Autodesk Inventor part; units mm, degrees
ref_plane "YZ Plane" through (0, 0, 0) normal (1, 0, 0) x (0, 1, 0)
ref_plane "XZ Plane" through (0, 0, 0) normal (0, 1, 0) x (-1, 0, 0)
ref_plane "XY Plane" through (0, 0, 0) normal (0, 0, 1) x (1, 0, 0)
sketch "Sketch1" plane through (0, 0, 0) normal (0, 0, 1) x (1, 0, 0)
  circle A0 centre (57.1655, 18.417) radius 2.1
  circle A1 centre (12.7885, 12.5269) radius 2.1
  circle A2 centre (17.2869, -26.8107) radius 2.1
  circle A3 centre (-1.1004, -6.0436) radius 5
  line L0 (64.4194, 6.1067) -> (62.3371, -1.6056)
  line L1 (67.3095, 9.3686) -> (64.4194, 6.1067)
  ellipse E0 centre (57.1655, 18.417) end of major axis (47.0979, 27.5508) minor radius 11.51 (67.3095, 9.3686) -> (68.6853, 21.7358) ccw
  ellipse E1 centre (54.4602, 15.4351) end of major axis (43.6731, 3.5452) minor radius 13.5934 (68.6853, 21.7358) -> (59.3507, 30.2045) ccw
  ellipse E2 centre (57.1655, 18.417) end of major axis (47.0979, 27.5508) minor radius 11.51 (59.3507, 30.2045) -> (47.0214, 27.4655) ccw
  line L2 (36.5043, 15.5956) -> (47.0214, 27.4655)
  arc A4 (36.5043, 15.5956) -> (29.6862, 12.4398) centre (33.7853, 12.5269) ccw
  line L3 (16.8875, 12.4398) -> (29.6862, 12.4398)
  arc A5 (16.8875, 12.4398) -> (10.0695, 15.5956) centre (12.7885, 12.5269) ccw
  line L4 (10.0695, 15.5956) -> (-0.4476, 27.4655)
  ellipse E3 centre (-10.5917, 18.417) end of major axis (-0.5241, 27.5508) minor radius 11.51 (-0.4476, 27.4655) -> (-12.7769, 30.2045) ccw
  ellipse E4 centre (-7.8864, 15.4351) end of major axis (2.9006, 3.5452) minor radius 13.5934 (-12.7769, 30.2045) -> (-22.1115, 21.7358) ccw
  ellipse E5 centre (-10.5917, 18.417) end of major axis (-0.5241, 27.5508) minor radius 11.51 (-22.1115, 21.7358) -> (-20.7358, 9.3686) ccw
  line L5 (-20.7358, 9.3686) -> (-17.8456, 6.1067)
  line L6 (-17.8456, 6.1067) -> (-15.7633, -1.6056)
  line L7 (-15.7633, -1.6056) -> (-6.4546, -11.2249)
  line L8 (-6.4546, -11.2249) -> (1.9738, -21.6241)
  line L9 (1.9738, -21.6241) -> (9.6038, -24.7107)
  line L10 (9.6038, -24.7107) -> (14.4693, -29.7892)
  arc A6 (14.4693, -29.7892) -> (17.2869, -30.9107) centre (17.2869, -26.8107) ccw
  line L11 (17.2869, -30.9107) -> (29.2869, -30.9107)
  arc A7 (29.2869, -30.9107) -> (32.1045, -29.7892) centre (29.2869, -26.8107) ccw
  line L12 (36.97, -24.7107) -> (32.1045, -29.7892)
  line L13 (44.6, -21.6241) -> (36.97, -24.7107)
  line L14 (53.0284, -11.2249) -> (44.6, -21.6241)
  line L15 (62.3371, -1.6056) -> (53.0284, -11.2249)
  circle A8 centre (-10.5917, 18.417) radius 2.1
  circle A9 centre (47.6742, -6.0436) radius 5
  circle A10 centre (29.2869, -26.8107) radius 2.1
  circle A11 centre (33.7853, 12.5269) radius 2.1
  arc A12 (-51.3703, 45.0767) -> (97.4441, 45.0767) centre (23.0369, 31.7099) ccw construction
  arc A13 (51.5869, 99.9923) -> (-5.5131, 99.9923) centre (23.0369, 31.7099) ccw construction
  arc A14 (-50.582, -28.3339) -> (101.2571, -22.203) centre (23.0369, 31.7099) ccw construction
  line L16 (23.0369, 31.7099) -> (23.2869, -30.9107) construction
  line L17 (85.5258, 132.2899) -> (-39.4742, 132.2899)
  line L18 (-39.4742, 132.2899) -> (-39.4742, -63.2901)
  line L19 (-39.4742, -63.2901) -> (85.5258, -63.2901)
  line L20 (85.5258, -63.2901) -> (85.5258, 132.2899)
  line L21 (85.5258, 132.2899) -> (-39.4742, -63.2901) construction
  line L22 (-39.4742, 132.2899) -> (85.5258, -63.2901) construction
  point P0 (0, 0)
  point P1 (23.0258, 34.4999)
  dimension "d0" = 195.58
  dimension "d27" = 125
extrude "Extrusion1" add sketch "Sketch1" along normal blind 4 contours L0 L15 L14 L13 L12 A7 L11 A6 L10 L9 L8 L7 L6 L5 E5 E4 E3 L4 A5 L3 A4 L2 E2 E1 E0 L1 | L20 L19 L18 L17
sketch "Sketch2" plane through (0, 0, 4) normal (0, 0, 1) x (1, 0, 0)
  line L0 (-39.4742, 132.2899) -> (-39.4742, -63.2901)
  line L1 (-39.4742, -63.2901) -> (85.5258, -63.2901)
  line L2 (85.5258, -63.2901) -> (85.5258, 132.2899)
  line L3 (85.5258, 132.2899) -> (-39.4742, 132.2899)
  circle A0 centre (12.7885, 12.5269) radius 2.1
  circle A1 centre (33.7853, 12.5269) radius 2.1
  circle A2 centre (29.2869, -26.8107) radius 2.1
  circle A3 centre (47.6742, -6.0436) radius 5
  circle A4 centre (-10.5917, 18.417) radius 2.1
  circle A5 centre (-1.1004, -6.0436) radius 5
  circle A6 centre (17.2869, -26.8107) radius 2.1
  circle A7 centre (57.1655, 18.417) radius 2.1
  line L4 (85.5258, 132.2899) -> (-39.4742, 132.2899)
  line L5 (-39.4742, 132.2899) -> (-39.4742, 127.2899)
  line L6 (-39.4742, 127.2899) -> (85.5258, 127.2899)
  line L7 (85.5258, 127.2899) -> (85.5258, 132.2899)
  line L8 (52.5258, 127.2899) -> (-6.4742, 127.2899)
  line L9 (-6.4742, 127.2899) -> (-6.4742, 133.2899)
  line L10 (-6.4742, 133.2899) -> (52.5258, 133.2899)
  line L11 (52.5258, 133.2899) -> (52.5258, 127.2899)
  point P0 (0, 0)
  point P1 (-39.4742, 127.2899)
  point P2 (85.5258, 127.2899)
  dimension "d3" = 5
  dimension "d7" = 6
  dimension "d8" = 33
  dimension "d9" = 33
extrude "Extrusion2" add sketch "Sketch2" along normal blind 130 contours L3 L9 L6 L0 | L3 L11 L6 L9 | L3 L2 L6 L11
sketch "Sketch4" plane through (0, 0, 134) normal (0, 0, 1) x (1, 0, 0)
  line L0 (85.5258, 127.2899) -> (-39.4742, 127.2899)
  line L1 (-39.4742, 127.2899) -> (-39.4742, -63.2901)
  line L2 (-39.4742, -63.2901) -> (85.5258, -63.2901)
  line L3 (85.5258, -63.2901) -> (85.5258, 127.2899)
  circle A0 centre (12.7885, 12.5269) radius 2.1
  circle A1 centre (33.7853, 12.5269) radius 2.1
  circle A2 centre (29.2869, -26.8107) radius 2.1
  circle A3 centre (47.6742, -6.0436) radius 5
  circle A4 centre (-10.5917, 18.417) radius 2.1
  circle A5 centre (-1.1004, -6.0436) radius 5
  circle A6 centre (17.2869, -26.8107) radius 2.1
  circle A7 centre (57.1655, 18.417) radius 2.1
  line L4 (85.5258, 127.2899) -> (85.5258, 132.2899)
  line L5 (85.5258, 132.2899) -> (-39.4742, 132.2899)
  line L6 (-39.4742, 132.2899) -> (-39.4742, 127.2899)
  line L7 (-39.4742, 127.2899) -> (85.5258, 127.2899)
  point P0 (0, 0)
extrude "Extrusion3" add sketch "Sketch4" along normal blind 4 contours L3 L2 L1 L0 | L0 L6 L5 L4 | A0 | A1 | A2 | A3 | A4 | A5 | A6 | A7
fillet "Fillet1" [suppressed]
sketch "Sketch6" plane through (0, 0, 138) normal (0, 0, 1) x (1, 0, 0)
  line L0 (85.5258, 132.2899) -> (-39.4742, 132.2899)
  line L1 (-39.4742, 132.2899) -> (-39.4742, -63.2901)
  line L2 (-39.4742, -63.2901) -> (85.5258, -63.2901)
  line L3 (85.5258, -63.2901) -> (85.5258, 132.2899)
  line L4 (48.5258, 138.9893) -> (-2.4742, 138.9893)
  line L5 (-2.4742, 138.9893) -> (-2.4742, 104.2541)
  line L6 (-2.4742, 104.2541) -> (48.5258, 104.2541)
  line L7 (48.5258, 104.2541) -> (48.5258, 138.9893)
  point P0 (0, 0)
  dimension "d16" = 37
  dimension "d17" = 37
extrude "Extrusion5" cut sketch "Sketch6" against normal blind 101.6 contours L7 L6 L5 L0 | L0 L5 L4 L7
fillet "Fillet2" radius 9.525 5 edges at (67.0258, 132.2899, 138) (-20.9742, 132.2899, 138) (23.0258, 132.2899, 0) (-20.9742, 127.2899, 134) (67.0258, 127.2899, 134)
chamfer "Chamfer1" distance 3.175 angle 45 8 edges at (23.0258, 132.2899, 36.4) (48.5258, 132.2899, 82.4375) (48.5258, 129.5001, 135.2102) (48.5258, 113.5095, 138) (-2.4742, 132.2899, 82.4375) (-2.4742, 129.5001, 135.2102) (-2.4742, 113.5095, 138) (23.0258, 104.2541, 138)
chamfer "Chamfer2" distance 4 angle 45 1 edges at (23.0258, 127.2899, 4)
equation "\"d9\" = d8"
equation "\"d17\" = d16"
properties part number "Head_Box_Base"
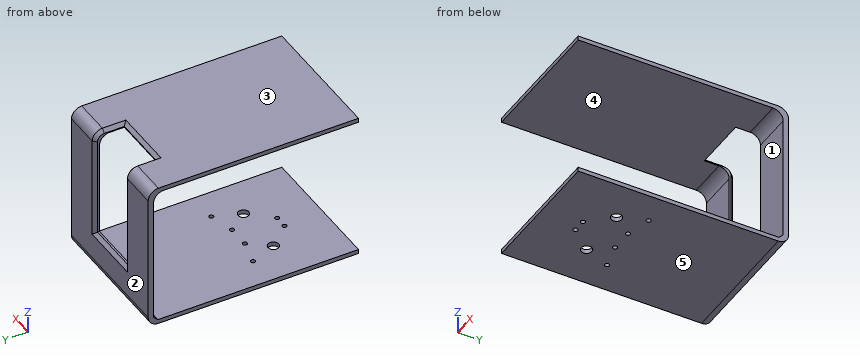
Source: CAD feature listing. Evaluate the final solid. Frame: model axes, mm. Face numbers are marked on the shaded views. A direction names the side the tool comes from. Round coordinates to 2 decimals unless told otherwise and drop trailing zeros. Order: outer loops, then holes, each group sorted by start corner. A loop starts at its lowest first (then second) coordinate and runs counter-clockwise, first axis right, second up. Notation, with made-up numbers: (12, -33.75) - (46, -33.75) arc R9 cw to (46, -26.75) - close; hole circle Ø10 at (65, -17.5). An arc over 180 degrees is marked (long way). Use a Markdown table: item, result. Add a question column.
1. Section query C-C (x = -26). Return the cut outline in (y, z) (3 decimals), then the cut area to 3 significant figures.
2. Section query B-B (y = 27). Return the cut outline in (x, z), then the cut area to 3 significant figures.
3. Line query: probe 1 along Z at (x, y) = (59.5, 48.5); probe 2 along Z at (x, y) = (-13, 123.5); probe 3 along Y at (x, z) = (10.5, 19). Output: solid intervals per line, ascending.
4. Mould query, pull axis Z, two halves, no side actions, for the marked faces 1, 2 and 3. Classes: +Z half, -Z half, draft (parallel to the pull), parting line (faces both ways), or undercut.
5. Section query A-A (z = 60). Return the cut outline in (x, y), then the cut area to 3 significant figures.
6. Set-up query: the marked faces 4 and 5. Return all of +Z, -Z, +X, -X, +Y, -Y with unobstructed straight access to the full face (end or side cutting, diameter ignored); none if empty.
7. First-contact query: pin 1 (5 mm diameter, centred on x = -13, z = 100.5, fed in from -Y); pin 2 (2.5 mm diameter, centred on x = -10.59, y = 18.42, fed in from -Z); pin 3 (0.9 mm diameter, centred on x = 20, z = 134.5, fed in from +Y). Flat tips, straight axial feed; report the tip coordinate or a pass-through.
Derived:
| question | item | result |
|---|---|---|
| 1 | outline | (-63.29, 0) - (122.765, 0) arc R9.525 ccw to (132.29, 9.525) - (132.29, 128.475) arc R9.525 ccw to (122.765, 138) - (-63.29, 138) - (-63.29, 134) - (117.765, 134) arc R9.525 cw to (127.29, 124.475) - (127.29, 8) - (123.29, 4) - (-63.29, 4) - close |
| 1 | area | 2,200 mm2 |
| 2 | outline | (-39.47, 0) - (85.53, 0) - (85.53, 4) - (-39.47, 4) - close; (-39.47, 134) - (85.53, 134) - (85.53, 138) - (-39.47, 138) - close |
| 2 | area | 1,000 mm2 |
| 3 | probe 1 | 0 to 4, 134 to 138 |
| 3 | probe 2 | 0.03 to 4.21, 132.08 to 137.97 |
| 3 | probe 3 | 127.29 to 132.29 |
| 4 | face 1 | undercut |
| 4 | face 2 | draft |
| 4 | face 3 | +Z half |
| 5 | outline | (-39.47, 127.29) - (-2.47, 127.29) - (-2.47, 129.11) - (-5.65, 132.29) - (-39.47, 132.29) - close; (48.53, 127.29) - (85.53, 127.29) - (85.53, 132.29) - (51.7, 132.29) - (48.53, 129.11) - close |
| 5 | area | 360 mm2 |
| 6 | face 4 | +X, -X, -Y |
| 6 | face 5 | -Z, +X, -X, +Y, -Y |
| 7 | pin 1 | y = 127.29 |
| 7 | pin 2 | z = 134 |
| 7 | pin 3 | y = 104.25 |
